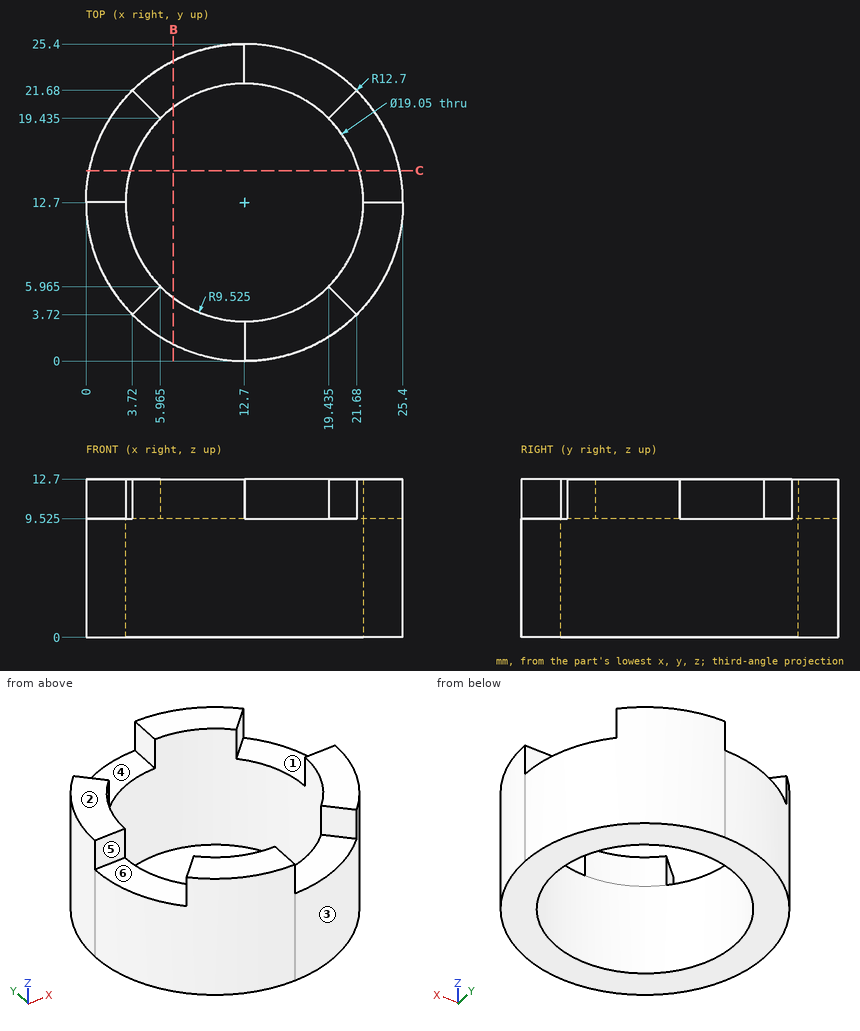
The figure shows three views and two pictorial views of one solid part (mm, origin at its lowest corner). Answer the questions. A direction names the side the tool comes from. Round coordinates to 2 decimals unless told otherwise and drop trailing zeros. Order: outer loops, then holes, each group sorted by start corner. A loop starts at its lowest first (then second) coordinate and runs counter-clockwise, first axis right, second up. Notation, with made-up numbers: (82, -8) - (87, -8) arc R21 cw to (87, 31) - close; hole circle Ø4 at (32.25, 39.5). An arc over 180 degrees is marked (long way). Write item = value, one per line. Start each with the question number.
1) Section C-C, the plane y = 15.25 is taken. Write down the section's boundary in (x, z) (1 decimal).
2) Straight lines are drawn through the part: L1, parallel to Y at x = 12.7, z = 3.25 (1 decimal); L2, parallel to Z at x = 19.5, y = 2.5 (1 decimal); L3, parallel to Y at x = 12.5, z = 11.5. For each, find the intervals that lie inside material, in ascending order.
3) Given pin 1 (1 mm diameter, centred on x = 24, z = 10.5, fed in from +Y); pin 2 (2.5 mm diameter, centred on y = 23.5, z = 12, fed in from -X); pin 3 (6.5 mm diameter, centred on x = 17.5, y = 3, fed in from +Z) (3 decimals); pin 4 (2 mm diameter, centred on x = 6, y = 11.5, fed in from -Z), each flat-ended and moving along its own axis, determine where each tip first touches the part or whether it passes through.
4) For a pull along Y with two mould halves and no side action, classify the marked faces 1, 2 and 3 as released by +Y, released by -Y, zero draft, split by the parting line, or undercut.
5) For the marked faces 4, 5 and 6, determine the directions among +Z, -Z, +X, -X, +Y, -Y from which every point of the face is accessible in a straight line to the end or side of a thin tool.
6) Section B-B, the plane x = 7 is taken. Write down the section's boundary in (y, z) (1 decimal).
Results list:
q1.outline = (0.3, 0) - (3.5, 0) - (3.5, 12.7) - (0.3, 12.7) - close; (21.9, 0) - (25.1, 0) - (25.1, 9.5) - (21.9, 9.5) - close
q2.L1 = 0 to 3.2, 22.2 to 25.4
q2.L2 = 0 to 9.5
q2.L3 = 0 to 3.18
q3.pin_1 = 12.7
q3.pin_2 = 12.7
q3.pin_3 = 9.525
q3.pin_4 = through
q4.face_1 = undercut
q4.face_2 = zero draft
q4.face_3 = released by -Y
q5.face_4 = +Z, +Y
q5.face_5 = +Z, -X, -Y
q5.face_6 = +Z, -X
q6.outline = (1.4, 0) - (5.1, 0) - (5.1, 12.7) - (1.4, 12.7) - close; (20.3, 0) - (24, 0) - (24, 9.5) - (20.3, 9.5) - close
